Geometry check sheet. Reference: the model listing, model coordinates, mm. A direction names the side the tool comes from. Coordinates: 2 decimals unless noted, no trailing zeros. Write each loop counter-clockwise with the first axis right and the second up, starting at its lowest first coordinate (ties: lowest second). Pieces come first, ordered by that corner, then holes. Notation, with made-up numbers: M 15,40 L 52,40 A23 cw 52,62 Z; hole C 39.5,-36.75 d10. An arc over 180 degrees is marked long. Answer as a JSON object with one key per item and string values. Group by question number.
```python
from build123d import *

# Parameters (mm, degrees)
EXTRUDE_1_DEPTH     = 7
SKETCH_2_R          = 2
CUT_EXTRUDE_1_DEPTH = 34.066457703


with BuildPart() as part:
    # 草图1 → 凸台-拉伸1 (new body)
    with BuildSketch(Plane.XY):
        Polygon((-2.375, -4), (-2.375, 11), (17.625, 11), (17.625, -4), (28.625, -4), (28.625, 0), (21.625, 0), (21.625, 15), (-6.375, 15), (-6.375, 0), (-13.375, 0), (-13.375, -4), align=None)
    extrude(amount=EXTRUDE_1_DEPTH)

    # 草图2 → 切除-拉伸1 (cut, through all)
    with BuildSketch(Plane(origin=(0, 0, 0), x_dir=(1, 0, 0), z_dir=(0, 1, 0))):
        with Locations(Location((25.125, -3.5, 0), (0, 0, 180))):
            Circle(SKETCH_2_R)
        with Locations((-9.875, -3.5)):
            Circle(SKETCH_2_R)
    extrude(amount=-CUT_EXTRUDE_1_DEPTH, mode=Mode.SUBTRACT)


solid = part.part
```
1) Section check A-A (z = 3.5). Record the cut outline in (x, y) (3 decimals), then the cut area to 3 significant figures.
2) Section check C-C (x = -9.5). Record the cut outline in (y, z).
3) Draft check along X on faces 5 (the flat face through (9, 13, 7)), 6 (the flat face through (21.625, 7, 3)), 7 (the cylindrical face through (27.123, -1.972, 3.588)). Enter one of: +X half, -X half, draft (parallel to the pull), parting line (faces both ways), or undercut.
4) Go/stop test with flat-tipped pins: pin 1 Ø3 at (x, y) = (22, 5.5) entering from +Z; pin 2 Ø3 at (x, z) = (-9.875, 3.5) entering from +Y; pin 3 Ø2 at (x, z) = (3.5, 5) entering from -Y; pin 4 Ø2 at (x, z) = (24, 4) entering from +Y. Record where each tip stops, or that it passes through.
5) Set-up check for faces 1 (the flat face through (27, 0, 5)), 2 (the flat face through (-13.375, -2, 3)), 3 (the flat face through (17.625, 4, 3)), 4 (the flat face through (-6.375, 8, 3)): record each of +Z, -Z, +X, -X, +Y, -Y from which the full face is reachable in a straight line by a thin tool's end or side.
6) Section check B-B (y = 4.25). Record the cut outline in (x, z) (3 decimals).
7) Section check D-D (z = 6). Record the cut outline in (x, y) (3 decimals), then the cut area to 3 significant figures.
8) Material ranges on probe 1 along X at (y, z) = (-2.5, 6) (3 decimals); probe 2 along X at (y, z) = (7.75, 1.5) (3 decimals); probe 3 along Y at (x, z) = (-11, 1), recorded low to high. Write a range as [from, to].
Entries:
{
 "1": {"outline": "M -13.375,-4 L -11.875,-4 L -11.875,0 L -13.375,0 Z; M -7.875,-4 L -2.375,-4 L -2.375,11 L 17.625,11 L 17.625,-4 L 23.125,-4 L 23.125,0 L 21.625,0 L 21.625,15 L -6.375,15 L -6.375,0 L -7.875,0 Z; M 27.125,-4 L 28.625,-4 L 28.625,0 L 27.125,0 Z", "area": "256 mm^2"},
 "2": {"outline": "M -4,0 L 0,0 L 0,1.54 L -4,1.54 Z; M -4,5.46 L 0,5.46 L 0,7 L -4,7 Z"},
 "3": {"face 5": "draft", "face 6": "+X half", "face 7": "undercut"},
 "4": {"pin 1": "z = 7", "pin 2": "through", "pin 3": "y = 11", "pin 4": "y = 0"},
 "5": {"face 1": "+Z, -Z, +X, +Y", "face 2": "+Z, -Z, -X, +Y, -Y", "face 3": "+Z, -Z, -Y", "face 4": "+Z, -Z, -X, +Y"},
 "6": {"outline": "M -6.375,0 L -2.375,0 L -2.375,7 L -6.375,7 Z; M 17.625,0 L 21.625,0 L 21.625,7 L 17.625,7 Z"},
 "7": {"outline": "M -13.375,-4 L -2.375,-4 L -2.375,11 L 17.625,11 L 17.625,-4 L 28.625,-4 L 28.625,0 L 21.625,0 L 21.625,15 L -6.375,15 L -6.375,0 L -13.375,0 Z", "area": "288 mm^2"},
 "8": {"probe 1": "[-13.375, -2.375], [17.625, 28.625]", "probe 2": "[-6.375, -2.375], [17.625, 21.625]", "probe 3": "[-4, 0]"}
}
